The model under review builds one solid part; all positions refer to its coordinate system, in mm. A direction names the side the tool comes from. Round coordinates to 2 decimals unless told otherwise and drop trailing zeros. Order: outer loops, then holes, each group sorted by start corner. A loop starts at its lowest first (then second) coordinate and runs counter-clockwise, first axis right, second up. Notation, with made-up numbers: M 88,-23 L 129,-23 A24 cw 129,1 Z; hole C -6,82 d2. An arc over 180 degrees is marked long. Use a Markdown table: item, result. Add a question column.
1. Consider section B-B on z = -6.5. State the section outline as (x, y) points, then the cut area to 3 significant figures.
2. The part is to be moulded in two halves that separate along Y. For faces 1 (the flat face through (25.413, -44.446, -39.376)), 2 (the cylindrical face through (9.4, -20.48, -39.41)), 3 (the cylindrical face through (9.4, -20.48, 39.38)), 4 (the flat face through (0, -2, 0)), say which applies: +Y half, -Y half, draft (parallel to the pull), parting line (faces both ways), or undercut.
3. Consider section A-A on x = 215.5. State the section outline as (y, z) points (3 decimals).
4. To check wall thickness, follow probe 1 along Z at (x, y) = (400.5, -37); probe 2 along Y at (x, z) = (120.5, 22). State the ranges of each line that lie inside material, in increasing order.
5. For faces 5 (the flat face through (221, -2.588, 0)), 6 (the flat face through (25.413, -44.446, 39.412)), list the 3-axis set-ups (+Z, -Z, +X, -X, +Y, -Y) from which the entire face can be reached by the end or side of a thin tool; tool diameter is ignored.
6. Insertion check: P1, Ø4, axis at x = 436.9, y = -13.36, coming from the -Z side; P2, Ø21, axis at x = 243.5, z = 6.5, coming from the -Y side. Each pin has a flat end and moves straight along its axis. Give the tip position at first contact, or say it passes through.
from build123d import *

# Parameters (mm, degrees)
BASE_FLANGE1_DEPTH           = 448.31
CUT_EXTRUDE1_DEPTH           = 459.458977562
F_1_4_CLEARANCE_HOLE1_D      = 7.2644
F_10_0_1935_DIAMETER_HOLE1_D = 4.9149
FILLET1_R                    = 3.81


# Sheet-metal steps are written as plain solids
with BuildPart() as part:
    # Sketch2 → Base-Flange1 (new body)
    with BuildSketch(Plane(origin=(0, 0, 0), x_dir=(0, 0, -1), z_dir=(1, 0, 0))):
        with BuildLine():
            Line((-40.68826, -50.8), (-40.68826, -5.76326))
            ThreePointArc((-40.68826, -5.76326), (-39.000240228, -1.688019772), (-34.925, 0))
            Line((-34.925, 0), (34.925, 0))
            ThreePointArc((34.925, 0), (39.000240228, -1.688019772), (40.68826, -5.76326))
            Line((40.68826, -5.76326), (40.68826, -50.8))
            Line((40.68826, -50.8), (38.1, -50.8))
            Line((38.1, -50.8), (38.1, -5.76326))
            ThreePointArc((38.1, -5.76326), (37.17006403, -3.51819597), (34.925, -2.58826))
            Line((34.925, -2.58826), (-34.925, -2.58826))
            ThreePointArc((-34.925, -2.58826), (-37.17006403, -3.51819597), (-38.1, -5.76326))
            Line((-38.1, -5.76326), (-38.1, -50.8))
            Line((-38.1, -50.8), (-40.68826, -50.8))
        make_face()
    extrude(amount=BASE_FLANGE1_DEPTH)

    # Sketch8 → Cut-Extrude1 (cut, through all)
    with BuildSketch(Plane.XY.offset(40.68826)):
        Polygon((0, -37.636171444), (49.128076995, -50.8), (0, -50.8), align=None)
    extrude(amount=-CUT_EXTRUDE1_DEPTH, mode=Mode.SUBTRACT)

    # 1/4 Clearance Hole1 (through all)
    with Locations(Plane.XY.offset(40.68826)):
        with Locations((8.61046841, -16.934326391)):
            Hole(F_1_4_CLEARANCE_HOLE1_D / 2)

    # #10 (0.1935) Diameter Hole1 (through all)
    with Locations(Plane.XY.offset(40.68826)):
        with Locations((410.50096824, -26.010505082), (413.952320207, -13.129884188), (436.899172539, -13.361871369), (431.968669729, -31.762758359), (39.880176489, -35.174025037), (45.632429766, -13.706323547), (85.501018246, -24.389079634), (134.570050222, -37.537087125)):
            Hole(F_10_0_1935_DIAMETER_HOLE1_D / 2)

    # Fillet1
    fillet1_edges = [part.edges().sort_by_distance(p)[0] for p in [
        (448.31, -50.8, 39.39413),
        (49.128076995, -50.8, -39.39413),
        (0, -37.636171444, -39.39413),
        (0, -37.636171444, 39.39413),
        (49.128076995, -50.8, 39.39413),
        (448.31, -50.8, -39.39413),
    ]]
    fillet(fillet1_edges, radius=FILLET1_R)


solid = part.part
Answer block:
| question | item | result |
|---|---|---|
| 1 | outline | M 0,-2.59 L 448.31,-2.59 L 448.31,0 L 0,0 Z |
| 1 | area | 1,160 mm^2 |
| 2 | face 1 | -Y half |
| 2 | face 2 | undercut |
| 2 | face 3 | undercut |
| 2 | face 4 | draft |
| 3 | outline | M -50.8,-40.688 L -5.763,-40.688 A5.763 ccw 0,-34.925 L 0,34.925 A5.763 ccw -5.763,40.688 L -50.8,40.688 L -50.8,38.1 L -5.763,38.1 A3.175 cw -2.588,34.925 L -2.588,-34.925 A3.175 cw -5.763,-38.1 L -50.8,-38.1 Z |
| 4 | probe 1 | -40.69 to -38.1, 38.1 to 40.69 |
| 4 | probe 2 | -2.59 to 0 |
| 5 | face 5 | +X, -X, -Y |
| 5 | face 6 | +Z, -Z, -X, -Y |
| 6 | P1 | through |
| 6 | P2 | y = -2.59 |
